Geometry: final body of the model. Coordinates: model frame, mm. A direction names the side the tool comes from. Coordinates: 2 decimals unless noted, no trailing zeros. Return JSON: item names as keys, results as strings.
from build123d import *

# Parameters (mm, degrees)
F0_R     = 9.5631
F1_DEPTH = 2.5
F2_R     = 1.729466
F3_DEPTH = 0.5
F4_R     = 4
F5_DEPTH = 3.5
F6_R     = 1.207107
F7_R     = 2
F8_DEPTH = 2.75
F9_R     = 0.482843
F10_R    = 0.458701


with BuildPart() as f1:
    # F0 (on Top) → F1 (new body)
    with BuildSketch(Plane.XY):
        Circle(F0_R)
    extrude(amount=F1_DEPTH)

    # F2 (on face) → F3 (cut)
    with BuildSketch(Plane.XY.offset(2.5)):
        with BuildLine():
            ThreePointArc((-7.558177, 0.272846), (-6.549837, 3.78155), (-4.01538, 6.40915))
            Line((-4.01538, 6.40915), (-4.515668, 7.275673))
            ThreePointArc((-4.515668, 7.275673), (-7.415862, 4.28155), (-8.558752, 0.272846))
            Line((-8.558752, 0.272846), (-7.558177, 0.272846))
        make_face()
        with BuildLine():
            ThreePointArc((-4.01538, 6.40915), (0, 7.5631), (4.01538, 6.40915))
            Line((4.01538, 6.40915), (4.515668, 7.275673))
            ThreePointArc((4.515668, 7.275673), (0, 8.5631), (-4.515668, 7.275673))
            Line((-4.515668, 7.275673), (-4.01538, 6.40915))
        make_face()
        with BuildLine():
            Line((4.515668, 7.275673), (4.01538, 6.40915))
            ThreePointArc((4.01538, 6.40915), (6.549837, 3.78155), (7.558177, 0.272846))
            Line((7.558177, 0.272846), (8.558752, 0.272846))
            ThreePointArc((8.558752, 0.272846), (7.415862, 4.28155), (4.515668, 7.275673))
        make_face()
        with BuildLine():
            Line((8.558752, 0.272846), (7.558177, 0.272846))
            ThreePointArc((7.558177, 0.272846), (7.561869, 0.136445), (7.5631, 0))
            ThreePointArc((7.5631, 0), (6.480548, -3.8991), (3.542796, -6.681996))
            Line((3.542796, -6.681996), (4.043084, -7.54852))
            ThreePointArc((4.043084, -7.54852), (7.3467, -4.399167), (8.5631, 0))
            ThreePointArc((8.5631, 0), (8.562013, 0.136441), (8.558752, 0.272846))
        make_face()
        with BuildLine():
            ThreePointArc((3.542796, -6.681996), (0, -7.5631), (-3.542796, -6.681996))
            Line((-3.542796, -6.681996), (-4.043084, -7.54852))
            ThreePointArc((-4.043084, -7.54852), (0, -8.5631), (4.043084, -7.54852))
            Line((4.043084, -7.54852), (3.542796, -6.681996))
        make_face()
        with BuildLine():
            ThreePointArc((-3.542796, -6.681996), (-6.549837, -3.78155), (-7.558177, 0.272846))
            Line((-7.558177, 0.272846), (-8.558752, 0.272846))
            ThreePointArc((-8.558752, 0.272846), (-7.415862, -4.28155), (-4.043084, -7.54852))
            Line((-4.043084, -7.54852), (-3.542796, -6.681996))
        make_face()
        with BuildLine():
            Line((4.01538, 6.40915), (1.594189, 2.215524))
            ThreePointArc((1.594189, 2.215524), (0, 2.729466), (-1.594189, 2.215524))
            Line((-1.594189, 2.215524), (-4.01538, 6.40915))
            ThreePointArc((-4.01538, 6.40915), (-6.549837, 3.78155), (-7.558177, 0.272846))
            Line((-7.558177, 0.272846), (-2.715795, 0.272846))
            ThreePointArc((-2.715795, 0.272846), (-2.363787, -1.364733), (-1.121605, -2.48837))
            Line((-1.121605, -2.48837), (-3.542796, -6.681996))
            ThreePointArc((-3.542796, -6.681996), (0, -7.5631), (3.542796, -6.681996))
            Line((3.542796, -6.681996), (1.121605, -2.48837))
            ThreePointArc((1.121605, -2.48837), (2.363787, -1.364733), (2.715795, 0.272846))
            Line((2.715795, 0.272846), (7.558177, 0.272846))
            ThreePointArc((7.558177, 0.272846), (6.549837, 3.78155), (4.01538, 6.40915))
        make_face()
        Circle(F2_R, mode=Mode.SUBTRACT)
    extrude(amount=-F3_DEPTH, mode=Mode.SUBTRACT)

    # F4 (on face) → F5 (join)
    with BuildSketch(Plane(origin=(0, 0, 0), x_dir=(1, 0, 0), z_dir=(0, 0, -1))):
        Circle(F4_R)
    extrude(amount=F5_DEPTH)

    # F6
    f6_edges = [f1.edges().sort_by_distance(p)[0] for p in [
        (-9.5631, 0, 0),
    ]]
    fillet(f6_edges, radius=F6_R)

    # F7 (on face) → F8 (join)
    with BuildSketch(Plane(origin=(0, 0, -3.5), x_dir=(1, 0, 0), z_dir=(0, 0, -1))):
        Circle(F7_R)
    extrude(amount=F8_DEPTH)

    # F9
    f9_edges = [f1.edges().sort_by_distance(p)[0] for p in [
        (-2, 0, -6.25),
    ]]
    fillet(f9_edges, radius=F9_R)

    # F10
    f10_edges = [f1.edges().sort_by_distance(p)[0] for p in [
        (-4, 0, -3.5),
    ]]
    fillet(f10_edges, radius=F10_R)


solid = f1.part
Item 1: First-contact query: pin 1 Ø3 at (x, y) = (5.5, 2.5) entering from -Z; pin 2 Ø5 at (x, z) = (5, -1) entering from +Y. Flat tips, straight axial feed; report the tip coordinate or a pass-through.
Worked out:
{"pin 1": "z = 0", "pin 2": "y = 8.91"}
Item 2: Reachability of faces 4 (the face through (-6.52, -3.83, 2.25)), 5 (the face through (2, 2, -3.5)), 6 (the face through (4, -2, 2.5)) from +Z, -Z, +X, -X, +Y, -Y: full face, straight path, thin tool, end or side. Return the list, or none.
Worked out:
{"face 4": "+Z", "face 5": "-Z", "face 6": "+Z, +X, -X, +Y, -Y"}
Item 3: Mould query, pull axis X, two halves, no side actions, for faces 1 (the face through (-4, -2, 2.5)), 2 (the face through (2.35, -1.39, 2.25)), 3 (the face through (0, 2, -5)). Classes: +X half, -X half, draft (parallel to the pull), parting line (faces both ways), or undercut.
Worked out:
{"face 1": "draft", "face 2": "undercut", "face 3": "parting line"}
Item 4: Ray query, probe 1 along X at (y, z) = (-4, 2.25); probe 2 along Z at (x, y) = (6.5, -4.75); probe 3 along Z at (x, y) = (-3.5, -4.25). Return the intervals inside material, ascending. Write a range as from..to.
Worked out:
{"probe 1": "-8.69..-7.57, -6.42..-1.99, 1.99..6.42, 7.57..8.69", "probe 2": "0..2", "probe 3": "0..2.5"}
